Source: CAD feature listing. Evaluate the final solid. Frame: model axes, mm. A direction names the side the tool comes from. Coordinates: 2 decimals unless noted, no trailing zeros. Write each loop counter-clockwise with the first axis right and the second up, starting at its lowest first coordinate (ties: lowest second). Pieces come first, ordered by that corner, then holes. Notation, with made-up numbers: (66, 37.5) -> (124, 37.5) arc R23 cw to (124, 75.5) -> close; hole circle Ø5 at (34, 36). An arc over 180 degrees is marked (long way). One line per item, written item: value. Start each with the question number.
1. First-contact query: P1, Ø1.5, axis at x = -23.5, z = 28, coming from the -Y side; P2, Ø1, axis at y = 22.5, z = 13.5, coming from the -X side. Flat tips, straight axial feed; report the tip coordinate or a pass-through.
2. Section query A-A, the plane x = -18.75. Output: boundary loops of the cut face in (y, z), and give its area (3 significant figures).
3. Section query C-C, the plane y = 20.5. Output: boundary loops of the cut face in (x, z).
4. Line query: line 1 (Y direction, x = -27.5, z = 26.5); line 2 (Z direction, x = -17, y = 18.5); line 3 (X direction, y = 19.75, z = 43). Output: solid intervals per line, ascending.
5. Section query B-B, the plane z = 38. Output: boundary loops of the cut face in (x, y), and give its area (3 significant figures).
6. Access query for faces 1 (the flat face through (-24, 19, 41)), 2 (the flat face through (-24, 23, 0)). Directions: +Z, -Z, +X, -X, +Y, -Y. A direction counts if a zero-diameter tool reaches every point of the face in a straight line with its end or side. Return the directions, or none.
from build123d import *

# Parameters (mm, degrees)
CROQUIS1_W              = 15
CROQUIS1_H              = 3.5
SALIENTE_EXTRUIR1_DEPTH = 41
SALIENTE_EXTRUIR3_DEPTH = 5


with BuildPart() as part:
    # Croquis1 → Saliente-Extruir1 (new body)
    with BuildSketch(Plane.XY):
        with Locations((-23.589562337, 23.303225109)):
            Rectangle(CROQUIS1_W, CROQUIS1_H)
    extrude(amount=SALIENTE_EXTRUIR1_DEPTH)

    # Croquis2 → Saliente-Extruir3 (add)
    with BuildSketch(Plane.XY.offset(41)):
        Polygon((-31.089562337, 25.053225109), (-31.101471771, 17.12903643), (-16.089562337, 17.12903643), (-16.089562337, 25.053225109), align=None)
    extrude(amount=SALIENTE_EXTRUIR3_DEPTH)


solid = part.part
Computed values:
1. P1: stops at y = 21.55
1. P2: stops at x = -31.09
2. outline: (17.13, 41) -> (21.55, 41) -> (21.55, 0) -> (25.05, 0) -> (25.05, 46) -> (17.13, 46) -> close
2. area: 183 mm²
3. outline: (-31.1, 41) -> (-16.09, 41) -> (-16.09, 46) -> (-31.1, 46) -> close
4. line 1: y = 21.55 to 25.05
4. line 2: z = 41 to 46
4. line 3: x = -31.1 to -16.09
5. outline: (-31.09, 21.55) -> (-16.09, 21.55) -> (-16.09, 25.05) -> (-31.09, 25.05) -> close
5. area: 52.5 mm²
6. face 1: -Z, +X, -X, -Y
6. face 2: -Z, +X, -X, +Y, -Y
